```python
from build123d import *

# Parameters (mm, degrees)
BOSS_EXTRUDE1_DEPTH        = 0.8
BOSS_EXTRUDE4_START        = -0.8
BOSS_EXTRUDE4_DEPTH        = 2.5
CUT_EXTRUDE2_DEPTH         = 1.5
M2_5_CLEARANCE_HOLE1_D     = 2.7
M2_5_CLEARANCE_HOLE1_DEPTH = 11.188838164
M2_5_CLEARANCE_HOLE1_TIP   = 0.811161836
BOSS_EXTRUDE7_START        = -1.5
SKETCH11_W                 = 1
SKETCH11_H                 = 1.5875
BOSS_EXTRUDE7_DEPTH        = 0.5
LPATTERN2_COUNT            = 10
LPATTERN2_PITCH            = 2
FILLET4_R                  = 8
FILLET6_SIZE               = 5
FILLET6_SIZE_2             = 10
FILLET7_SIZE               = 5
FILLET7_SIZE_2             = 10


with BuildPart() as part:
    # Sketch3 → Boss-Extrude1 (new body)
    with BuildSketch(Plane(origin=(0, 0, 0), x_dir=(1, 0, 0), z_dir=(0, 1, 0))):
        with BuildLine():
            ThreePointArc((-8.964400592, 29.591990842), (0, 30.92), (8.964400592, 29.591990842))
            ThreePointArc((8.964400592, 29.591990842), (12.633049801, 26.719344266), (13.403780114, 22.124014011))
            ThreePointArc((13.403780114, 22.124014011), (12.736333478, 19.347857063), (11.892930693, 16.62))
            Line((11.892930693, 16.62), (16.263283948, 16.62))
            Line((16.263283948, 16.62), (16.263283948, 42.786292272))
            Line((16.263283948, 42.786292272), (-16.835608917, 42.786292272))
            Line((-16.835608917, 42.786292272), (-16.835608917, 16.62))
            Line((-16.835608917, 16.62), (-11.892930693, 16.62))
            ThreePointArc((-11.892930693, 16.62), (-12.736333478, 19.347857063), (-13.403780114, 22.124014011))
            ThreePointArc((-13.403780114, 22.124014011), (-12.633049801, 26.719344266), (-8.964400592, 29.591990842))
        make_face()
        with BuildLine():
            Line((-10.5, 32.42), (16.263283948, 32.42))
            Line((16.263283948, 32.42), (16.263283948, 34.0075))
            Line((16.263283948, 34.0075), (-10.5, 34.0075))
            ThreePointArc((-10.5, 34.0075), (-11.207106781, 34.300393219), (-11.5, 35.0075))
            Line((-11.5, 35.0075), (-11.5, 38.0075))
            ThreePointArc((-11.5, 38.0075), (-11.207106781, 38.714606781), (-10.5, 39.0075))
            Line((-10.5, 39.0075), (16.263283948, 39.0075))
            Line((16.263283948, 39.0075), (16.263283948, 40.595))
            Line((16.263283948, 40.595), (-10.5, 40.595))
            ThreePointArc((-10.5, 40.595), (-12.329638796, 39.837138796), (-13.0875, 38.0075))
            Line((-13.0875, 38.0075), (-13.0875, 35.0075))
            ThreePointArc((-13.0875, 35.0075), (-12.329638796, 33.177861204), (-10.5, 32.42))
        make_face()
        with BuildLine():
            Line((-10.5, 34.0075), (16.263283948, 34.0075))
            Line((16.263283948, 34.0075), (16.263283948, 39.0075))
            Line((16.263283948, 39.0075), (-10.5, 39.0075))
            ThreePointArc((-10.5, 39.0075), (-11.207106781, 38.714606781), (-11.5, 38.0075))
            Line((-11.5, 38.0075), (-11.5, 35.0075))
            ThreePointArc((-11.5, 35.0075), (-11.207106781, 34.300393219), (-10.5, 34.0075))
        make_face()
    extrude(amount=-BOSS_EXTRUDE1_DEPTH)

    # Sketch3<5> → Boss-Extrude4 (add)
    with BuildSketch(Plane(origin=(0, 0, 0), x_dir=(1, 0, 0), z_dir=(0, 1, 0)).offset(BOSS_EXTRUDE4_START)):
        with BuildLine():
            ThreePointArc((-8.964400592, 29.591990842), (0, 30.92), (8.964400592, 29.591990842))
            ThreePointArc((8.964400592, 29.591990842), (12.633049801, 26.719344266), (13.403780114, 22.124014011))
            ThreePointArc((13.403780114, 22.124014011), (12.736333478, 19.347857063), (11.892930693, 16.62))
            Line((11.892930693, 16.62), (16.263283948, 16.62))
            Line((16.263283948, 16.62), (16.263283948, 42.786292272))
            Line((16.263283948, 42.786292272), (-16.835608917, 42.786292272))
            Line((-16.835608917, 42.786292272), (-16.835608917, 16.62))
            Line((-16.835608917, 16.62), (-11.892930693, 16.62))
            ThreePointArc((-11.892930693, 16.62), (-12.736333478, 19.347857063), (-13.403780114, 22.124014011))
            ThreePointArc((-13.403780114, 22.124014011), (-12.633049801, 26.719344266), (-8.964400592, 29.591990842))
        make_face()
        with BuildLine():
            ThreePointArc((8.964400592, 29.591990842), (12.633049801, 26.719344266), (13.403780114, 22.124014011))
            ThreePointArc((13.403780114, 22.124014011), (12.736333478, 19.347857063), (11.892930693, 16.62))
            Line((11.892930693, 16.62), (-11.892930693, 16.62))
            ThreePointArc((-11.892930693, 16.62), (-12.736333478, 19.347857063), (-13.403780114, 22.124014011))
            ThreePointArc((-13.403780114, 22.124014011), (-12.633049801, 26.719344266), (-8.964400592, 29.591990842))
            ThreePointArc((-8.964400592, 29.591990842), (0, 30.92), (8.964400592, 29.591990842))
        make_face()
        with BuildLine():
            Line((-10.5, 32.42), (16.263283948, 32.42))
            Line((16.263283948, 32.42), (16.263283948, 34.0075))
            Line((16.263283948, 34.0075), (-10.5, 34.0075))
            ThreePointArc((-10.5, 34.0075), (-11.207106781, 34.300393219), (-11.5, 35.0075))
            Line((-11.5, 35.0075), (-11.5, 38.0075))
            ThreePointArc((-11.5, 38.0075), (-11.207106781, 38.714606781), (-10.5, 39.0075))
            Line((-10.5, 39.0075), (16.263283948, 39.0075))
            Line((16.263283948, 39.0075), (16.263283948, 40.595))
            Line((16.263283948, 40.595), (-10.5, 40.595))
            ThreePointArc((-10.5, 40.595), (-12.329638796, 39.837138796), (-13.0875, 38.0075))
            Line((-13.0875, 38.0075), (-13.0875, 35.0075))
            ThreePointArc((-13.0875, 35.0075), (-12.329638796, 33.177861204), (-10.5, 32.42))
        make_face()
        with BuildLine():
            Line((-10.5, 34.0075), (16.263283948, 34.0075))
            Line((16.263283948, 34.0075), (16.263283948, 39.0075))
            Line((16.263283948, 39.0075), (-10.5, 39.0075))
            ThreePointArc((-10.5, 39.0075), (-11.207106781, 38.714606781), (-11.5, 38.0075))
            Line((-11.5, 38.0075), (-11.5, 35.0075))
            ThreePointArc((-11.5, 35.0075), (-11.207106781, 34.300393219), (-10.5, 34.0075))
        make_face()
    extrude(amount=-BOSS_EXTRUDE4_DEPTH)

    # Sketch3<7> → Cut-Extrude2 (cut)
    with BuildSketch(Plane(origin=(0, 0, 0), x_dir=(1, 0, 0), z_dir=(0, 1, 0))):
        with BuildLine():
            Line((-10.5, 32.42), (16.263283948, 32.42))
            Line((16.263283948, 32.42), (16.263283948, 34.0075))
            Line((16.263283948, 34.0075), (-10.5, 34.0075))
            ThreePointArc((-10.5, 34.0075), (-11.207106781, 34.300393219), (-11.5, 35.0075))
            Line((-11.5, 35.0075), (-11.5, 38.0075))
            ThreePointArc((-11.5, 38.0075), (-11.207106781, 38.714606781), (-10.5, 39.0075))
            Line((-10.5, 39.0075), (16.263283948, 39.0075))
            Line((16.263283948, 39.0075), (16.263283948, 40.595))
            Line((16.263283948, 40.595), (-10.5, 40.595))
            ThreePointArc((-10.5, 40.595), (-12.329638796, 39.837138796), (-13.0875, 38.0075))
            Line((-13.0875, 38.0075), (-13.0875, 35.0075))
            ThreePointArc((-13.0875, 35.0075), (-12.329638796, 33.177861204), (-10.5, 32.42))
        make_face()
    extrude(amount=-CUT_EXTRUDE2_DEPTH, mode=Mode.SUBTRACT)

    # M2.5 Clearance Hole1
    with Locations(Plane(origin=(0, 0, 0), x_dir=(1, 0, 0), z_dir=(0, 1, 0))):
        with Locations((-9, 36.5075), (9, 36.5075)):
            Hole(M2_5_CLEARANCE_HOLE1_D / 2, depth=M2_5_CLEARANCE_HOLE1_DEPTH)
            with Locations((0, 0, -(M2_5_CLEARANCE_HOLE1_DEPTH + M2_5_CLEARANCE_HOLE1_TIP / 2))):  # 118° drill point
                Cone(0, M2_5_CLEARANCE_HOLE1_D / 2, M2_5_CLEARANCE_HOLE1_TIP, mode=Mode.SUBTRACT)

    # Sketch11 → Boss-Extrude7 (add)
    with BuildSketch(Plane(origin=(0, 0, 0), x_dir=(1, 0, 0), z_dir=(0, 1, 0)).offset(BOSS_EXTRUDE7_START)):
        with Locations((10.763283948, 39.80125)):
            Rectangle(SKETCH11_W, SKETCH11_H)
        with Locations((10.763283948, 33.21375)):
            Rectangle(SKETCH11_W, SKETCH11_H)
    boss_extrude7 = extrude(amount=BOSS_EXTRUDE7_DEPTH)

    # LPattern2: Boss-Extrude7 ×10
    with Locations(*[(-i * LPATTERN2_PITCH, 0, 0) for i in range(1, LPATTERN2_COUNT)]):
        add(boss_extrude7)

    # Fillet4
    fillet4_edges = [part.edges().sort_by_distance(p)[0] for p in [
        (16.263283948, -1.65, -42.786292272),
        (-16.835608917, -1.65, -42.786292272),
    ]]
    fillet(fillet4_edges, radius=FILLET4_R)

    # Fillet6
    # an asymmetric fillet: 10, 5 mm, written as the material it takes off along each edge
    with BuildSketch(Plane(origin=(16.263283948, -28.3, -16.62), x_dir=(-1, 0, 0), z_dir=(0, 1, 0))) as fillet6_piece_1:
        with BuildLine():
            Bezier((FILLET6_SIZE, 0), (0, 0), (0, -FILLET6_SIZE_2), weights=[1, 0.707106781, 1])
            Line((0, -FILLET6_SIZE_2), (0, 0))
            Line((0, 0), (FILLET6_SIZE, 0))
        make_face()
    extrude(amount=53.3, mode=Mode.SUBTRACT)

    # Fillet7
    # an asymmetric fillet: 10, 5 mm, written as the material it takes off along each edge
    with BuildSketch(Plane(origin=(-16.835608917, 25, -16.62), x_dir=(1, 0, 0), z_dir=(0, -1, 0))) as fillet7_piece_1:
        with BuildLine():
            Bezier((FILLET7_SIZE, 0), (0, 0), (0, -FILLET7_SIZE_2), weights=[1, 0.707106781, 1])
            Line((0, -FILLET7_SIZE_2), (0, 0))
            Line((0, 0), (FILLET7_SIZE, 0))
        make_face()
    extrude(amount=53.3, mode=Mode.SUBTRACT)


solid = part.part
```
Can you work these out from the model? Positions are in its coordinate system, mm. A direction names the side the tool comes from. Round coordinates to 2 decimals unless told otherwise and drop trailing zeros. Loops run counter-clockwise (first coordinate to the right, second up) from the corner with the lowest first, then second, coordinate; pieces in that order, holes last.
Item 1: Please list where these lines run through material, in increasing order: L1, parallel to Z at x = 5, y = -0.25 (1 decimal); L2, parallel to Z at x = -10.5, y = -0.25 (1 decimal); L3, parallel to Z at x = -9, y = -1.7.
Item 2: Will these pins go through, and if not, where does the flat tip stop? pin 1 Ø0.8 at (x, z) = (8, -40) entering from +Y; pin 2 Ø0.5 at (x, z) = (13, -33) entering from +Y; pin 3 Ø1 at (y, z) = (-1.5, -38.5) entering from +X.
Item 3: Suppose I cut it at B-B, the plane y = -2.65. State how many separate pieces and enclosed holes the cut face has, then the cut area to 3 significant figures.
Item 4: Suppose I cut it at A-A, the plane z = -37. Write out the boundary of the cut face in (x, y).
Item 5: Which directions (+Z, -Z, +X, -X, +Y, -Y) give clear straight access to the entire face, cutting with the end or side of a thin tool? Please do faces 1 (the cylindrical face through (13.858, -1.673, -40.505)), 2 (the cylindrical face through (-12.726, -0.394, -19.31)), 3 (the flat face through (14, -1.5, -33)).
Item 6: If we mould it in two halves opening along Z, with no side actions, what happens to faces 4 (the flat face through (10, -1.5, -33)), 5 (the flat face through (-16.836, -2, -31)), 6 (the flat face through (0, -2, -16.62)), 7 (the flat face through (7, -1, -33))? For each: +Z half, -Z half, draft (parallel to the pull), parting line (faces both ways), or undercut.
Reported:
1. L1: z = -42.8 to -40.6, -39 to -34, -32.4 to -30.5
1. L2: z = -42.6 to -40.6, -39 to -34, -32.4 to -28.9
1. L3: z = -42.78 to -37.86, -35.16 to -16.62
2. pin 1: stops at y = -1
2. pin 2: stops at y = -1.5
2. pin 3: stops at x = 15.59
3. separate pieces: 1
3. enclosed holes: 2
3. area: 806 mm2
4. outline: (-16.52, -3.3) - (-10.26, -3.3) - (-10.26, 0) - (-11.5, 0) - (-11.5, -1.5) - (-13.09, -1.5) - (-13.09, 0) - (-16.52, 0) - close; (-7.74, -3.3) - (7.74, -3.3) - (7.74, 0) - (-7.74, 0) - close; (10.26, -3.3) - (15.95, -3.3) - (15.95, 0) - (10.26, 0) - close
5. face 1: -Z, +X, +Y, -Y
5. face 2: +Y
5. face 3: +X, +Y
6. face 4: undercut
6. face 5: draft
6. face 6: +Z half
6. face 7: undercut
